For this review, use the dimensioned drawing (mm, ordinates from the lowest corner) and the shaded views. A direction names the side the tool comes from. Coordinates: 2 decimals unless noted, no trailing zeros. Write each loop counter-clockwise with the first axis right and the second up, starting at its lowest first coordinate (ties: lowest second). Pieces come first, ordered by that corner, then holes. Notation, with made-up numbers: M 56,-17 L 97,-17 A10 cw 97,-4 Z; hole C -6,12.25 d11. An arc over 180 degrees is marked long. One line per question, with ' | ' between items.
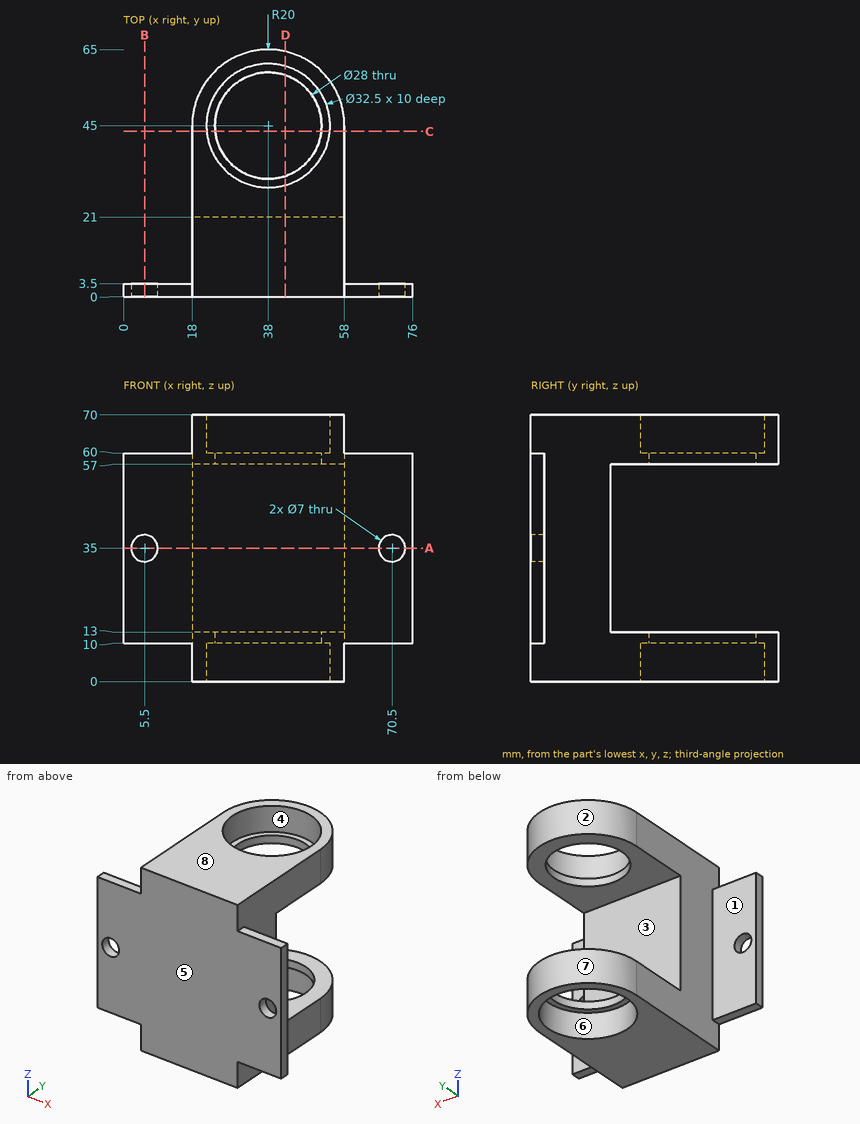
1. Take a section at C-C (y = 43.5). Write out the cut boundary in (x, z).
Answer sheet:
outline: M 18,0 L 21.82,0 L 21.82,10 L 24.08,10 L 24.08,13 L 18,13 Z; M 18,57 L 24.08,57 L 24.08,60 L 21.82,60 L 21.82,70 L 18,70 Z; M 51.92,10 L 54.18,10 L 54.18,0 L 58,0 L 58,13 L 51.92,13 Z; M 51.92,57 L 58,57 L 58,70 L 54.18,70 L 54.18,60 L 51.92,60 Z
2. Take a section at B-B (x = 5.5). Write out the cut boundary in (y, z).
Answer sheet:
outline: M 0,10 L 3.5,10 L 3.5,31.5 L 0,31.5 Z; M 0,38.5 L 3.5,38.5 L 3.5,60 L 0,60 Z
3. Take a section at A-A (z = 35). Write out the cut boundary in (x, y), then the cut area to 3 significant figures.
Answer sheet:
outline: M 0,0 L 2,0 L 2,3.5 L 0,3.5 Z; M 9,0 L 67,0 L 67,3.5 L 58,3.5 L 58,21 L 18,21 L 18,3.5 L 9,3.5 Z; M 74,0 L 76,0 L 76,3.5 L 74,3.5 Z | area: 917 mm^2
4. Insertion check: pin 1 Ø4 at (y, z) = (18, 31.5) entering from -X; pin 2 Ø25 at (x, y) = (38, 45) entering from +Z (1 decimal); pin 3 Ø5 at (y, z) = (16.5, 18.5) entering from +X; pin 4 Ø14.5 at (x, z) = (12, 36.5) entering from +Y. Each pin has a flat end and moves straight along its axis. Give the tip position at first contact, or say it passes through.
Answer sheet:
pin 1: x = 18 | pin 2: through | pin 3: x = 58 | pin 4: y = 21
5. Draft analysis for pull direction X (two halves, no side actions). For the marked faces 6, 7 and 8, state which applies: pulls with the +X half, pulls with the -X half, needs draft (parallel to the pull), parting line crosses it, or undercut.
Answer sheet:
face 6: undercut | face 7: parting line crosses it | face 8: needs draft
6. To check wall thickness, follow line 1 along Y through (x, z) = (38, 62); line 2 along Z through (x, y) = (35, 24); line 3 along Y through (x, z) = (54, 56). State the ranges of each line that lie inside material, in increasing order. Write a range as [from, to].
Answer sheet:
line 1: [0, 28.75], [61.25, 65] | line 2: [0, 13], [57, 70] | line 3: [0, 21]
7. Take a section at D-D (x = 42.5). Write out the cut boundary in (y, z), then the cut area to 3 significant figures.
Answer sheet:
outline: M 0,0 L 29.39,0 L 29.39,10 L 31.74,10 L 31.74,13 L 21,13 L 21,57 L 31.74,57 L 31.74,60 L 29.39,60 L 29.39,70 L 0,70 Z; M 58.26,10 L 60.61,10 L 60.61,0 L 64.49,0 L 64.49,13 L 58.26,13 Z; M 58.26,57 L 64.49,57 L 64.49,70 L 60.61,70 L 60.61,60 L 58.26,60 Z | area: 1,820 mm^2
8. Tool access review of the marked faces 1, 2, 3, 4 and 5: name each direction out of +Z, -Z, +X, -X, +Y, -Y from which nothing blocks a thin tool from reaching the whole face with its end or side.
Answer sheet:
face 1: +Z, -Z, -X, +Y | face 2: +Z, -Z, +Y | face 3: +X, -X, +Y | face 4: +Z | face 5: +Z, -Z, +X, -X, -Y
